from build123d import *

# Parameters (mm, degrees)
CYLINDER001_R     = 2
CYLINDER001_DEPTH = 4
CYLINDER_R        = 2
CYLINDER_DEPTH    = 4
BOX003_W          = 2
BOX003_H          = 30
BOX003_DEPTH      = 20
FILLET_R          = 3
BOX002_W          = 30
BOX002_H          = 40
BOX002_DEPTH      = 2.4
BOX001_W          = 30
BOX001_H          = 20
BOX001_DEPTH      = 2.4
BOX_W             = 50
BOX_H             = 100
BOX_DEPTH         = 2
FILLET002_R       = 3
FILLET003_R       = 2
CYLINDER003_R     = 2
CYLINDER003_DEPTH = 4
CYLINDER002_R     = 2
CYLINDER002_DEPTH = 4
BOX004_W          = 2
BOX004_H          = 30
BOX004_DEPTH      = 20
FILLET001_R       = 3
FILLET004_R       = 2


with BuildPart() as cylinder001:
    # Cylinder001 → Cylinder001 (new body)
    with BuildSketch(Plane(origin=(-3, 23, 11), x_dir=(0, 0, -1), z_dir=(1, 0, 0))):
        Circle(CYLINDER001_R)
    extrude(amount=CYLINDER001_DEPTH)


with BuildPart() as fusion001:
    # Cylinder → Cylinder (new body)
    with BuildSketch(Plane(origin=(-3, 7, 11), x_dir=(0, 0, -1), z_dir=(1, 0, 0))):
        Circle(CYLINDER_R)
    extrude(amount=CYLINDER_DEPTH)

    # Fusion001: union Cylinder001
    add(cylinder001.part)


with BuildPart() as obj1:
    # Box003 → Box003 (new body)
    with BuildSketch(Plane(origin=(-2, 0, 0), x_dir=(1, 0, 0), z_dir=(0, 0, 1))):
        with Locations((1, 15)):
            Rectangle(BOX003_W, BOX003_H)
    extrude(amount=BOX003_DEPTH)

    # Cut001: cut Fusion001
    add(fusion001.part, mode=Mode.SUBTRACT)

    # Fillet
    fillet_edges = [obj1.edges().sort_by_distance(p)[0] for p in [
        (-1, 0, 20),
        (-1, 30, 20),
    ]]
    fillet(fillet_edges, radius=FILLET_R)


with BuildPart() as hueco_inferior_40x30:
    # Box002 → Box002 (new body)
    with BuildSketch(Plane(origin=(10, 10, -0.2), x_dir=(1, 0, 0), z_dir=(0, 0, 1))):
        with Locations((15, 20)):
            Rectangle(BOX002_W, BOX002_H)
    extrude(amount=BOX002_DEPTH)


with BuildPart() as huecos_base:
    # Box001 → Box001 (new body)
    with BuildSketch(Plane(origin=(10, 70, -0.2), x_dir=(1, 0, 0), z_dir=(0, 0, 1))):
        with Locations((15, 10)):
            Rectangle(BOX001_W, BOX001_H)
    extrude(amount=BOX001_DEPTH)

    # Fusion: union hueco_inferior_40x30
    add(hueco_inferior_40x30.part)


with BuildPart() as obj2:
    # Box → Box (new body)
    with BuildSketch(Plane.XY):
        with Locations((25, 50)):
            Rectangle(BOX_W, BOX_H)
    extrude(amount=BOX_DEPTH)

    # Cut: cut huecos_base
    add(huecos_base.part, mode=Mode.SUBTRACT)

    # Fillet002
    fillet002_edges = [obj2.edges().sort_by_distance(p)[0] for p in [
        (40, 70, 1),
        (10, 70, 1),
        (40, 90, 1),
        (10, 90, 1),
        (40, 10, 1),
        (10, 10, 1),
        (40, 50, 1),
        (10, 50, 1),
    ]]
    fillet(fillet002_edges, radius=FILLET002_R)

    # Fillet003
    fillet003_edges = [obj2.edges().sort_by_distance(p)[0] for p in [
        (0, 100, 1),
        (50, 100, 1),
    ]]
    fillet(fillet003_edges, radius=FILLET003_R)


with BuildPart() as cylinder003:
    # Cylinder003 → Cylinder003 (new body)
    with BuildSketch(Plane(origin=(-3, 23, 11), x_dir=(0, 0, -1), z_dir=(1, 0, 0))):
        Circle(CYLINDER003_R)
    extrude(amount=CYLINDER003_DEPTH)


with BuildPart() as fusion002:
    # Cylinder002 → Cylinder002 (new body)
    with BuildSketch(Plane(origin=(-3, 7, 11), x_dir=(0, 0, -1), z_dir=(1, 0, 0))):
        Circle(CYLINDER002_R)
    extrude(amount=CYLINDER002_DEPTH)

    # Fusion002: union Cylinder003
    add(cylinder003.part)


with BuildPart() as pieza_final:
    # Box004 → Box004 (new body)
    with BuildSketch(Plane(origin=(-2, 0, 0), x_dir=(1, 0, 0), z_dir=(0, 0, 1))):
        with Locations((1, 15)):
            Rectangle(BOX004_W, BOX004_H)
    extrude(amount=BOX004_DEPTH)

    # Cut002: cut Fusion002
    add(fusion002.part, mode=Mode.SUBTRACT)

    # Fillet001
    fillet001_edges = [pieza_final.edges().sort_by_distance(p)[0] for p in [
        (-1, 0, 20),
        (-1, 30, 20),
    ]]
    fillet(fillet001_edges, radius=FILLET001_R)


with BuildPart() as pieza_final_1:
    # Fillet001 placement: moved
    add(pieza_final.part.moved(Location((52, 0, 0))))

    # Fusion003: union obj1, obj2
    add(obj1.part)
    add(obj2.part)

    # Fillet004
    fillet004_edges = [pieza_final_1.edges().sort_by_distance(p)[0] for p in [
        (52, 15, 0),
        (-2, 15, 0),
    ]]
    fillet(fillet004_edges, radius=FILLET004_R)


solid = pieza_final_1.part
For this review, take the finished solid that the model builds, in its own axes (mm). A direction names the side the tool comes from. Round coordinates to 2 decimals unless told otherwise and drop trailing zeros. Loops run counter-clockwise (first coordinate to the right, second up) from the corner with the lowest first, then second, coordinate; pieces in that order, holes last. Notation, with made-up numbers: (51, 27) - (91, 27) arc R12 cw to (91, 37) - close; hole circle Ø9 at (41.25, 87.5). An arc over 180 degrees is marked (long way). Put each result on its own line as item: value. Start each with the question number.
1. Consider section B-B on z = 6.75. State the section outline as (x, y) points, plus the area to 3 significant figures.
2. Consider section D-D on x = 29.5. State the section outline as (y, z) points, plus the area to 3 significant figures.
3. For faces 1 (the flat face through (10, 30, 1)), 2 (the flat face through (50, 15, 11)), 3 (the cylindrical face through (-0.99, 0.86, 19.1)), list the 3-axis set-ups (+Z, -Z, +X, -X, +Y, -Y) from which the entire face can be reached by the end or side of a thin tool; tool diameter is ignored.
4. Insertion check: P1, Ø1, axis at y = 78.5, z = 1, coming from the +X side; P2, Ø1.6, axis at y = 25, z = 0.5, coming from the +X side; P3, Ø8, axis at x = 39, y = 54, coming from the +Z side. Each pin has a flat end and moves straight along its axis. Give the tip position at first contact, or say it passes through.
5. Mouldability with a two-part tool opening along X and no side actions: class faces 4 (the cylindrical face through (10.86, 49.1, 1.01)), 5 (the cylindrical face through (-1.4, 15.21, 0.57)), 6 (the cylindrical face through (-0.99, 29.1, 19.14)) as +X half, -X half, draft (parallel to the pull), parting line (faces both ways), or undercut.
6. Consider section A-A on y = 7. State the section outline as (x, z) points.
7. Consider section C-C on y = 84.5. State the section outline as (x, z) points, plus the area to 3 significant figures.
8. For probe 1 along Y at (x, z) = (50.9, 11); probe 2 along X at (y, z) = (13, 17); probe 3 along Z at (x, y) = (11, 6.5), list the stretches that pass through material, from the lowest coordinate up. Write a range as [from, to].
Result sheet:
1. outline: (-2, 0) - (0, 0) - (0, 30) - (-2, 30) - close; (50, 0) - (52, 0) - (52, 30) - (50, 30) - close
1. area: 120 mm^2
2. outline: (0, 0) - (10, 0) - (10, 2) - (0, 2) - close; (50, 0) - (70, 0) - (70, 2) - (50, 2) - close; (90, 0) - (100, 0) - (100, 2) - (90, 2) - close
2. area: 80.0 mm^2
3. face 1: +Z, -Z
3. face 2: +Z, +Y, -Y
3. face 3: +Z, +X, -X, -Y
4. P1: x = 50
4. P2: x = 51.87
4. P3: z = 2
5. face 4: undercut
5. face 5: -X half
5. face 6: draft
6. outline: (-2, 2) arc R2 ccw to (0, 0) - (50, 0) arc R2 ccw to (52, 2) - (52, 9) - (50, 9) - (50, 2) - (0, 2) - (0, 9) - (-2, 9) - close; (-2, 13) - (0, 13) - (0, 20) - (-2, 20) - close; (50, 13) - (52, 13) - (52, 20) - (50, 20) - close
7. outline: (0, 0) - (10, 0) - (10, 2) - (0, 2) - close; (40, 0) - (50, 0) - (50, 2) - (40, 2) - close
7. area: 40.0 mm^2
8. probe 1: [0, 5], [9, 21], [25, 30]
8. probe 2: [-2, 0], [50, 52]
8. probe 3: [0, 2]
